```python
from build123d import *

# Parameters (mm, degrees)
F0_R     = 200
F1_DEPTH = 520
F0_R_2   = 50
F0_W     = 120
F0_H     = 280
F2_DEPTH = 120
F0_R_3   = 100
F3_DEPTH = 120
F5_DEPTH = 100
F6_R     = 110
F7_DEPTH = 289.1810463391


with BuildPart() as f1:
    # F0 (on Front) → F1 (new body)
    with BuildSketch(Plane.XZ):
        with BuildLine():
            Line((-60, 280), (60, 280))
            Line((60, 280), (550, 280))
            Line((550, 280), (550, 415))
            Line((550, 415), (394.6834174373, 415))
            ThreePointArc((394.6834174373, 415), (341.3155900504, 439.7023731306), (325.6138193858, 496.375))
            ThreePointArc((325.6138193858, 496.375), (321.7066673274, 623.5174822551), (270, 739.7366596101))
            Line((270, 739.7366596101), (270, 936.2514615059))
            Line((270, 936.2514615059), (270, 996.2514615059))
            Line((270, 996.2514615059), (-270, 996.2514615059))
            Line((-270, 996.2514615059), (-270, 936.2514615059))
            Line((-270, 936.2514615059), (-270, 739.7366596101))
            ThreePointArc((-270, 739.7366596101), (-321.7066673274, 623.5174822551), (-325.6138193858, 496.375))
            ThreePointArc((-325.6138193858, 496.375), (-341.3155900504, 439.7023731306), (-394.6834174373, 415))
            Line((-394.6834174373, 415), (-550, 415))
            Line((-550, 415), (-550, 280))
            Line((-550, 280), (-60, 280))
        make_face()
        with Locations((0, 550)):
            Circle(F0_R, mode=Mode.SUBTRACT)
    extrude(amount=F1_DEPTH)

    # F0 (on Front) → F2 (join)
    with BuildSketch(Plane.XZ):
        with BuildLine():
            Line((60, 0), (450, 0))
            ThreePointArc((450, 0), (520.7106781187, 29.2893218813), (550, 100))
            Line((550, 100), (550, 280))
            Line((550, 280), (60, 280))
            Line((60, 280), (60, 0))
        make_face()
        with Locations((450, 100)):
            Circle(F0_R_2, mode=Mode.SUBTRACT)
        with Locations((0, 140)):
            Rectangle(F0_W, F0_H)
        with BuildLine():
            Line((-60, 280), (60, 280))
            Line((60, 280), (550, 280))
            Line((550, 280), (550, 415))
            Line((550, 415), (394.6834174373, 415))
            ThreePointArc((394.6834174373, 415), (341.3155900504, 439.7023731306), (325.6138193858, 496.375))
            ThreePointArc((325.6138193858, 496.375), (321.7066673274, 623.5174822551), (270, 739.7366596101))
            Line((270, 739.7366596101), (270, 936.2514615059))
            Line((270, 936.2514615059), (270, 996.2514615059))
            Line((270, 996.2514615059), (-270, 996.2514615059))
            Line((-270, 996.2514615059), (-270, 936.2514615059))
            Line((-270, 936.2514615059), (-270, 739.7366596101))
            ThreePointArc((-270, 739.7366596101), (-321.7066673274, 623.5174822551), (-325.6138193858, 496.375))
            ThreePointArc((-325.6138193858, 496.375), (-341.3155900504, 439.7023731306), (-394.6834174373, 415))
            Line((-394.6834174373, 415), (-550, 415))
            Line((-550, 415), (-550, 280))
            Line((-550, 280), (-60, 280))
        make_face()
        with Locations((0, 550)):
            Circle(F0_R, mode=Mode.SUBTRACT)
        with BuildLine():
            Line((-450, 0), (-60, 0))
            Line((-60, 0), (-60, 280))
            Line((-60, 280), (-550, 280))
            Line((-550, 280), (-550, 100))
            ThreePointArc((-550, 100), (-520.7106781187, 29.2893218813), (-450, 0))
        make_face()
        with Locations((-450, 100)):
            Circle(F0_R_2, mode=Mode.SUBTRACT)
        with BuildLine():
            Line((394.6834174373, 415), (550, 415))
            Line((550, 415), (270, 936.2514615059))
            Line((270, 936.2514615059), (270, 739.7366596101))
            ThreePointArc((270, 739.7366596101), (321.7066673274, 623.5174822551), (325.6138193858, 496.375))
            ThreePointArc((325.6138193858, 496.375), (341.3155900504, 439.7023731306), (394.6834174373, 415))
        make_face()
        with BuildLine():
            Line((-270, 936.2514615059), (-550, 415))
            Line((-550, 415), (-394.6834174373, 415))
            ThreePointArc((-394.6834174373, 415), (-341.3155900504, 439.7023731306), (-325.6138193858, 496.375))
            ThreePointArc((-325.6138193858, 496.375), (-321.7066673274, 623.5174822551), (-270, 739.7366596101))
            Line((-270, 739.7366596101), (-270, 936.2514615059))
        make_face()
        with BuildLine():
            Line((-270, 996.2514615059), (270, 996.2514615059))
            Line((270, 996.2514615059), (270, 1106.2514615059))
            ThreePointArc((270, 1106.2514615059), (240.7106781187, 1176.9621396245), (170, 1206.2514615059))
            Line((170, 1206.2514615059), (-170, 1206.2514615059))
            ThreePointArc((-170, 1206.2514615059), (-240.7106781187, 1176.9621396245), (-270, 1106.2514615059))
            Line((-270, 1106.2514615059), (-270, 996.2514615059))
        make_face()
        with Locations((-170, 1106.2514615059)):
            Circle(F0_R_2, mode=Mode.SUBTRACT)
        with Locations((170, 1106.2514615059)):
            Circle(F0_R_2, mode=Mode.SUBTRACT)
    extrude(amount=F2_DEPTH)

    # F0 (on Front) → F3 (join)
    with BuildSketch(Plane.XZ):
        with Locations((0, 550)):
            Circle(F0_R)
        with Locations((0, 550)):
            Circle(F0_R_3, mode=Mode.SUBTRACT)
    extrude(amount=F3_DEPTH)

    # F4 (on face) → F5 (cut)
    with BuildSketch(Plane.XY.offset(996.2514615059)):
        with BuildLine():
            ThreePointArc((146.1913956702, -320), (99.32848066, -206.8629150102), (-13.8086043298, -160))
            Line((-13.8086043298, -160), (-13.8086043298, -210))
            ThreePointArc((-13.8086043298, -210), (63.9731416007, -242.2182540695), (96.1913956702, -320))
            ThreePointArc((96.1913956702, -320), (63.9731416007, -397.7817459305), (-13.8086043298, -430))
            Line((-13.8086043298, -430), (-13.8086043298, -480))
            ThreePointArc((-13.8086043298, -480), (99.32848066, -433.1370849898), (146.1913956702, -320))
        make_face()
        with BuildLine():
            Line((-13.8086043298, -210), (-13.8086043298, -160))
            ThreePointArc((-13.8086043298, -160), (-173.8086043298, -320), (-13.8086043298, -480))
            Line((-13.8086043298, -480), (-13.8086043298, -430))
            ThreePointArc((-13.8086043298, -430), (-123.8086043298, -320), (-13.8086043298, -210))
        make_face()
    extrude(amount=-F5_DEPTH, mode=Mode.SUBTRACT)

    # F6 (on face) → F7 (cut, through all)
    with BuildSketch(Plane.XY.offset(996.2514615059)):
        with Locations((-13.8086043298, -320)):
            Circle(F6_R)
    extrude(amount=-F7_DEPTH, mode=Mode.SUBTRACT)


solid = f1.part
```
Input: part model. Units: mm. Frame: model coordinates. A direction names the side the tool comes from. Round coordinates to 2 decimals unless told otherwise and drop trailing zeros. Write each loop counter-clockwise with the first axis right and the second up, starting at its lowest first coordinate (ties: lowest second). Pieces come first, ordered by that corner, then holes. Notation, with made-up numbers: M 45,47 L 63,47 A17 ccw 63,75 Z; hole C 0,79.25 d10. An arc over 180 degrees is marked long. Write each question's results on one line, items separated by ' | '.
Q1. Section query A-A (x = -144.5). Return loops of the section in (y, z), and give its area (3 significant figures).
Results:
outline: M -520,280 L -120,280 L -120,0 L 0,0 L 0,1063.24 L -120,1063.24 L -120,996.25 L -227.7,996.25 L -227.7,896.25 L -412.3,896.25 L -412.3,996.25 L -520,996.25 L -520,688.27 L -120,688.27 L -120,411.73 L -520,411.73 Z; M -120,1149.26 L 0,1149.26 L 0,1206.25 L -120,1206.25 Z | area: 292,000 mm^2
Q2. Draft query along Z for faces 1 (the face through (-321.303, -317.2, 625.263)), 2 (the face through (411.96, -59.16, 671.98)), 3 (the face through (-270, -256, 885)). Return one class per face: released by +Z, released by -Z, zero draft, split by the parting line, or undercut.
Results:
face 1: undercut | face 2: released by +Z | face 3: zero draft
Q3. Access query for faces 4 (the face through (42, -120, 642)), 5 (the face through (124, -228, 996.251)), 6 (the face through (341.87, -317.2, 439.06)). Directions: +Z, -Z, +X, -X, +Y, -Y. A direction counts if a zero-diameter tool reaches every point of the face in a straight line with its end or side. Return the directions, or none.
Results:
face 4: -Y | face 5: +Z, +X, -X, -Y | face 6: +X, -Y
Q4. Section query D-D (x = 0). Return loops of the section in (y, z), and give its area (3 significant figures).
Results:
outline: M -520,280 L -120,280 L -120,0 L 0,0 L 0,450 L -120,450 L -120,350 L -520,350 Z; M -520,750 L -429.13,750 L -429.13,896.25 L -479.4,896.25 L -479.4,996.25 L -520,996.25 Z; M -210.87,750 L -120,750 L -120,650 L 0,650 L 0,1206.25 L -120,1206.25 L -120,996.25 L -160.6,996.25 L -160.6,896.25 L -210.87,896.25 Z | area: 183,000 mm^2
Q5. Line query: line 1 along Z through (x, y) = (0, -65); line 2 along Z through (x, y) = (-170, -42.5); line 3 along X through (y, z) = (-95, 141). Output: solid intervals per line, ascending.
Results:
line 1: z = 0 to 450, 650 to 1206.25 | line 2: z = 0 to 1056.25, 1156.25 to 1206.25 | line 3: x = -550 to -478.62, -421.38 to 421.38, 478.62 to 550
Q6. Section query B-B (y = -140). Return loops of the section in (x, z) (3 decimals).
Results:
outline: M -550,280 L 550,280 L 550,415 L 394.683,415 A70 cw 325.614,496.375 A330 ccw 270,739.737 L 270,996.251 L -270,996.251 L -270,739.737 A330 ccw -325.614,496.375 A70 cw -394.683,415 L -550,415 Z; hole C 0,550 d400
Q7. Section query C-C (z = 550). Return loops of the section in (x, y), and give its area (3 significant figures).
Results:
outline: M -477.48,-120 L -330,-120 L -330,-520 L -200,-520 L -200,-120 L -100,-120 L -100,0 L -477.48,0 Z; M 100,-120 L 200,-120 L 200,-520 L 330,-520 L 330,-120 L 477.48,-120 L 477.48,0 L 100,0 Z | area: 195,000 mm^2
Q8. Pin query (flat end, axial travel): P1, Ø3, axis at x = -229.5, y = -194, coming from the -Z side; P2, Ø1, axis at x = 380.5, y = -175.5, coming from the +Z side; P3, Ø10, axis at x = 233, z = 1082, coming from the +Y side; P4, Ø3, axis at y = -330, z = 912.5, coming from the +X side. Return the tip coordinate at first contact, or that it passes through.
Results:
P1: stops at z = 280 | P2: stops at z = 416.56 | P3: stops at y = 0 | P4: stops at x = 270
